Autodesk Inventor part; units mm, degrees
ref_plane "YZ Plane" through (0, 0, 0) normal (1, 0, 0) x (0, 1, 0)
ref_plane "XZ Plane" through (0, 0, 0) normal (0, 1, 0) x (-1, 0, 0)
ref_plane "XY Plane" through (0, 0, 0) normal (0, 0, 1) x (1, 0, 0)
sketch "Sketch1" plane through (0, 0, 0) normal (0, 1, 0) x (-1, 0, 0)
  circle A0 centre (0, 0) radius 9.525
  dimension "d0" = 19.05
extrude "Extrusion1" add sketch "Sketch1" along normal mid plane 127
sketch "Sketch2" plane through (0, 63.5, 0) normal (0, 1, 0) x (1, 0, 0)
  circle A0 centre (0, 0) radius 9.525
  circle A1 centre (0, 0) radius 4.7625
  dimension "d3" = 9.525
  dimension "d4" = 19.05
extrude "Extrusion2" cut sketch "Sketch2" against normal blind 15.875
sketch "Sketch3" plane through (0, -63.5, 0) normal (0, -1, 0) x (1, 0, 0)
  circle A0 centre (0, 0) radius 4.7625
  circle A1 centre (0, 0) radius 9.525
  dimension "d7" = 9.525
extrude "Extrusion3" cut sketch "Sketch3" against normal blind 15.875
properties part number "drum" material "Aluminum 6061"
Geometry check sheet. Reference: the model listing, model coordinates, mm. A direction names the side the tool comes from. Round coordinates to 2 decimals unless told otherwise and drop trailing zeros. Loops run counter-clockwise (first coordinate to the right, second up) from the corner with the lowest first, then second, coordinate; pieces in that order, holes last. Notation, with made-up numbers: (6, -9) - (52, -9) arc R25 ccw to (52, 20) - close; hole circle Ø6 at (42.25, 75). An arc over 180 degrees is marked (long way). One line per question, with ' | ' between items. Start each with the question number.
1. Scan lines: line 1 (Y direction, x = -4.5, z = -4) (3 decimals); line 2 (Z direction, x = -0.5, y = -15); line 3 (X direction, y = -47, z = 8.25). Record each from-to range of solid material in increasing order. Write a range as [from, to].
2. Cross-section at B-B on z = 0. Record the cut outline in (x, y) (1 decimal), then the cut area to 3 significant figures.
3. Cross-section at A-A on x = 0. Record the cut outline in (y, z) (1 decimal), then the cut area to 3 significant figures.
4. Depth check by flat-ended pin: pin 1 (3 mm diameter, centred on x = -1.5, y = 21, fed in from -Z) (3 decimals); pin 2 (1 mm diameter, centred on y = 49.5, z = 3.5, fed in from +X); pin 3 (1.5 mm diameter, centred on y = 15.5, z = 7, fed in from +X). Enter the tip coordinate at first touch or a pass-through.
5. Cross-section at D-D on x = 8. Record the cut outline in (y, z) (3 decimals).
6. Cross-section at C-C on y = -6. Record the cut outline in (x, z) (3 decimals).
7. Tool access check on faces 1 (the face through (-2.3, 47.625, -4.4)), 2 (the face through (-3.78, -55.67, -2.9)), 3 (the face through (0, -63.5, 0)). Record the directions out of +Z, -Z, +X, -X, +Y, -Y that give a thin tool (end or side, any length) a straight path to the whole face; none if there is none.
Taken from the geometry:
1) line 1: [-47.625, 47.625] | line 2: [-9.51, 9.51] | line 3: [-4.76, 4.76]
2) outline: (-9.5, -47.6) - (-4.8, -47.6) - (-4.8, -63.5) - (4.8, -63.5) - (4.8, -47.6) - (9.5, -47.6) - (9.5, 47.6) - (4.8, 47.6) - (4.8, 63.5) - (-4.8, 63.5) - (-4.8, 47.6) - (-9.5, 47.6) - close | area: 2,120 mm²
3) outline: (-63.5, -4.8) - (-47.6, -4.8) - (-47.6, -9.5) - (47.6, -9.5) - (47.6, -4.8) - (63.5, -4.8) - (63.5, 4.8) - (47.6, 4.8) - (47.6, 9.5) - (-47.6, 9.5) - (-47.6, 4.8) - (-63.5, 4.8) - close | area: 2,120 mm²
4) pin 1: z = -9.525 | pin 2: x = 3.7 | pin 3: x = 7.19
5) outline: (-47.625, -5.17) - (47.625, -5.17) - (47.625, 5.17) - (-47.625, 5.17) - close
6) outline: circle Ø19.05 at (0, 0)
7) face 1: +Y | face 2: -Y | face 3: +Z, -Z, +X, -X, -Y
